Model file for the job. Use its own axes, mm. A direction names the side the tool comes from. Coordinates: 2 decimals unless noted, no trailing zeros. Order: outer loops, then holes, each group sorted by start corner. A loop starts at its lowest first (then second) coordinate and runs counter-clockwise, first axis right, second up. Notation, with made-up numbers: (44.5, 2) -> (66.5, 2) arc R17 ccw to (66.5, 29) -> close; hole circle Ø10 at (51.25, -3.5). An arc over 180 degrees is marked (long way). Use CSV: the item, a comma, the result in double quotes. Start each with the question number.
(1) Probe L1, parallel to Y at x = 0, z = 3.8; L2, parallel to Y at x = -1, z = 13.25; L3, parallel to Z at x = 29, y = -53. List the from-to ranges inside material, lowest first.
(2) Cut at B-B on x = -58. Write the cut outline in (y, z).
(3) Pull direction Z, two halves, no side cores. Call faces 3 (the cylindrical face through (-55.69, -0.96, 2.46)), 4 (the flat face through (29, 1, 0)), 5 (the cylindrical face through (44.746, -46.512, 9.945)), 6 (the cylindrical face through (-45.104, 46.054, 8.946)): pulls with the +Z half, pulls with the -Z half, needs draft (parallel to the pull), parting line crosses it, or undercut.
(4) Cut at A-A on y = 0. Write the cut outline in (x, z).
(5) Cut at D-D on x = -39. Write the cut outline in (y, z).
(6) Tool access for faces 1 (the cylindrical face through (1.34, -55.89, 2.46)), 2 (the cylindrical face through (-8.071, 61.472, 9.93)): list every direction of +Z, -Z, +X, -X, +Y, -Y with a clear straight run to the whole face (end or side of a thin tool).
(7) Pin check, flat tips, straight feed: pin 1 Ø4 at (x, z) = (-51, 3.5) entering from +Y; pin 2 Ø8 at (x, z) = (-38.5, 2.5) entering from -Y; pin 3 Ø3 at (x, z) = (-48.5, 5) entering from -Y. Stop position of each tip, or through.
```python
from build123d import *

# Parameters (mm, degrees)
SKETCH1_R               = 67
SKETCH1_R_2             = 2.5
BOSS_EXTRUDE1_DEPTH     = 5
SKETCH3_R               = 25
CUT_EXTRUDE1_DEPTH      = 10
SKETCH4_R               = 67
SKETCH4_R_2             = 62
BOSS_EXTRUDE2_DEPTH     = 10
CUT_EXTRUDE4_DEPTH      = 121
CUT_EXTRUDE4_DEPTH_BACK = 121
SKETCH7_R               = 1.25


with BuildPart() as part:
    # Sketch1 → Boss-Extrude1 (new body)
    with BuildSketch(Plane.XY):
        Circle(SKETCH1_R)
        with Locations((0, 58)):
            Circle(SKETCH1_R_2, mode=Mode.SUBTRACT)
        with Locations((58, 0)):
            Circle(SKETCH1_R_2, mode=Mode.SUBTRACT)
        with Locations((0, -58)):
            Circle(SKETCH1_R_2, mode=Mode.SUBTRACT)
        with Locations((-58, 0)):
            Circle(SKETCH1_R_2, mode=Mode.SUBTRACT)
    extrude(amount=BOSS_EXTRUDE1_DEPTH)

    # Sketch3 → Cut-Extrude1 (cut)
    with BuildSketch(Plane.XY.offset(5)):
        Circle(SKETCH3_R)
    extrude(amount=-CUT_EXTRUDE1_DEPTH, mode=Mode.SUBTRACT)

    # Sketch4 → Boss-Extrude2 (add)
    with BuildSketch(Plane.XY.offset(5)):
        Circle(SKETCH4_R)
        Circle(SKETCH4_R_2, mode=Mode.SUBTRACT)
    extrude(amount=BOSS_EXTRUDE2_DEPTH)

    # Sketch7 → Cut-Extrude4 (cut, two sides: drawn at the far end of the back side and taken through both)
    with BuildSketch(Plane(origin=(0, 0, 0), x_dir=(0.7071067811865477, 0.7071067811865475, 0), z_dir=(-0.7071067811865475, 0.7071067811865477, 0)).offset(-CUT_EXTRUDE4_DEPTH_BACK)):
        with Locations((0, -10)):
            Circle(SKETCH7_R)
    extrude(amount=CUT_EXTRUDE4_DEPTH + CUT_EXTRUDE4_DEPTH_BACK, mode=Mode.SUBTRACT)


solid = part.part
```
Outcome:
1,L1,"-67 to -60.5, -55.5 to -25, 25 to 55.5, 60.5 to 67"
1,L2,"-66.99 to -61.99, 61.99 to 66.99"
1,L3,"0 to 5"
2,outline,"(-33.54, 0) -> (-2.5, 0) -> (-2.5, 5) -> (-21.91, 5) -> (-21.91, 15) -> (-33.54, 15) -> close; (2.5, 0) -> (33.54, 0) -> (33.54, 15) -> (21.91, 15) -> (21.91, 5) -> (2.5, 5) -> close"
3,face 3,"needs draft"
3,face 4,"pulls with the -Z half"
3,face 5,"undercut"
3,face 6,"undercut"
4,outline,"(-67, 0) -> (-60.5, 0) -> (-60.5, 5) -> (-62, 5) -> (-62, 15) -> (-67, 15) -> close; (-55.5, 0) -> (-25, 0) -> (-25, 5) -> (-55.5, 5) -> close; (25, 0) -> (55.5, 0) -> (55.5, 5) -> (25, 5) -> close; (60.5, 0) -> (67, 0) -> (67, 15) -> (62, 15) -> (62, 5) -> (60.5, 5) -> close"
5,outline,"(-54.48, 0) -> (54.48, 0) -> (54.48, 15) -> (48.2, 15) -> (48.2, 5) -> (-48.2, 5) -> (-48.2, 15) -> (-54.48, 15) -> close"
6,face 1,"+Z, -Z"
6,face 2,"+Z"
7,pin 1,"y = 45.69"
7,pin 2,"y = -57.43"
7,pin 3,"y = -47.75"
